Geometry: see drawing. Coordinates: mm, zero at the bounding-box minimum. A direction names the side the tool comes from. Coordinates: 2 decimals unless noted, no trailing zeros. Use a Markdown table: item, result. Add a question column.
Q1. Section query A-A (z = 34.5). Give the number of separate pieces and of enclosed holes in the cut face.
Q2. Pin query (flat end, axial travel): P1, Ø1.4, axis at x = 31, z = 22.5, coming from the -Y side (1 decimal); P2, Ø10, axis at x = 13, z = 50.5, coming from the -Y side (1 decimal); P3, Ø1.5, axis at x = 28.5, y = 64, coming from the +Z side (1 decimal). Return the tip coordinate at first contact, or that it passes through.
Q3. Material intervals for probe 1 along X at (y, z) = (100, 64.5) (1 decimal); probe 2 along Y at (x, z) = (49.5, 6); probe 3 along X at (y, z) = (35, 33.5), sorted ascending. Write a range as from..to.
Q4. Mould query, pull axis X, two halves, no side actions, for the marked faces 6, 7, 8 and 9. Classes: released by +X, released by -X, zero draft, split by the parting line, or undercut.
Q5. Set-up query: the marked faces 1, 2, 3, 4 and 5. Return all of +Z, -Z, +X, -X, +Y, -Y with unobstructed straight access to the full face (end or side cutting, diameter ignored); none if empty.
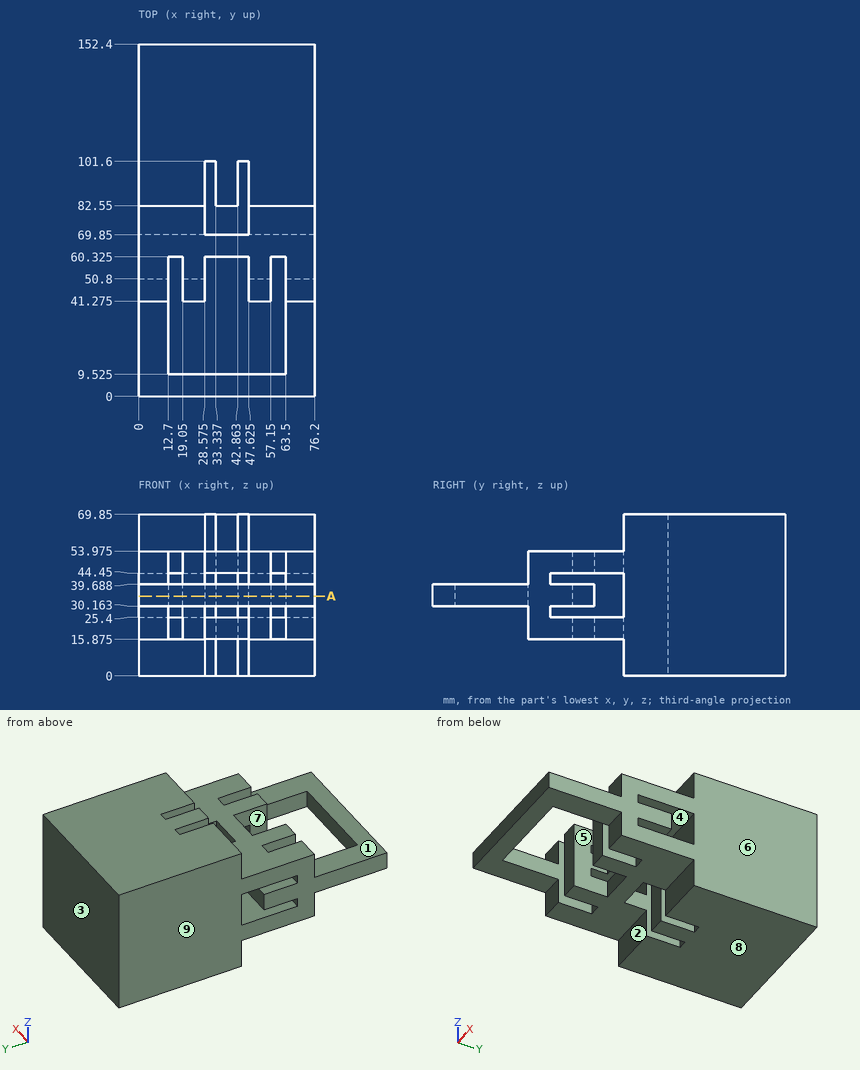
Values follow:
| question | item | result |
|---|---|---|
| 1 | separate pieces | 2 |
| 1 | enclosed holes | 1 |
| 2 | P1 | y = 60.3 |
| 2 | P2 | y = 41.3 |
| 2 | P3 | z = 54 |
| 3 | probe 1 | 0..28.6, 33.3..42.9, 47.6..76.2 |
| 3 | probe 2 | 82.55..152.4 |
| 3 | probe 3 | 0..12.7, 63.5..76.2 |
| 4 | face 6 | released by +X |
| 4 | face 7 | undercut |
| 4 | face 8 | zero draft |
| 4 | face 9 | released by -X |
| 5 | face 1 | +Z, +X, -X, -Y |
| 5 | face 2 | -Z, +X, -X, -Y |
| 5 | face 3 | +Z, -Z, +X, -X, +Y |
| 5 | face 4 | +X, -X |
| 5 | face 5 | +Z, -Z |
